from build123d import *

# Parameters (mm, degrees)
SKETCH_1_W      = 200
SKETCH_1_H      = 200
EXTRUDE_1_DEPTH = 150
SKETCH_2_R      = 40
EXTRUDE_2_DEPTH = 10
EXTRUDE_START   = 10
SKETCH_3_R      = 40
EXTRUDE_3_DEPTH = 10


with BuildPart() as part:
    # 草图1 → 凸台-拉伸1 (new, symmetric)
    with BuildSketch(Plane.XY):
        Rectangle(SKETCH_1_W, SKETCH_1_H)
    extrude(amount=EXTRUDE_1_DEPTH, both=True)

    # 草图2 → 凸台-拉伸2 (add)
    with BuildSketch(Plane.XY.offset(150)):
        Circle(SKETCH_2_R)
    extrude(amount=EXTRUDE_2_DEPTH)

    # 草图3 → 凸台-拉伸3 (add)
    with BuildSketch(Plane(origin=(0, 0, -150), x_dir=(-1, 0, 0), z_dir=(0, 0, -1)).offset(EXTRUDE_START)):
        with Locations(Location((0, 0, 0), (0, 0, 180))):
            Circle(SKETCH_3_R)
    extrude(amount=-EXTRUDE_3_DEPTH)


solid = part.part
Design review of the part built by this model. Coordinates are the model's own, in mm. A direction names the side the tool comes from. Round coordinates to 2 decimals unless told otherwise and drop trailing zeros. Write each loop counter-clockwise with the first axis right and the second up, starting at its lowest first coordinate (ties: lowest second). Pieces come first, ordered by that corner, then holes. Notation, with made-up numbers: (-31, 36.5) - (-14, 36.5) arc R9 ccw to (-14, 47.5) - close; hole circle Ø8 at (46.5, 69). An arc over 180 degrees is marked (long way). Use a Markdown table: item, result. Add a question column.
1. We need section C-C (x = 51.5). State the section outline as (y, z) points.
2. For faces 1 (the face through (-1, 46, -150)), 2 (the face through (-1, -1, -160)), 3 (the face through (-8.67, -39.05, 154.93)), list the 3-axis set-ups (+Z, -Z, +X, -X, +Y, -Y) from which the entire face can be reached by the end or side of a thin tool; tool diameter is ignored.
3. Clearance check with flat-ended pins moving along their axes: pin 1 (12 mm diameter, centred on x = 10.5, y = 60, fed in from -Z); pin 2 (1.5 mm diameter, centred on x = -47, y = 58.5, fed in from +Z). State where each tip first meets the part, or that it passes through.
4. We need section A-A (x = 0). State the section outline as (y, z) points.
5. Wall thickness on probe 1 along Z at (x, y) = (69, -30.5): over which ranges is the line inside the solid? List them lowest first.
Output:
| question | item | result |
|---|---|---|
| 1 | outline | (-100, -150) - (100, -150) - (100, 150) - (-100, 150) - close |
| 2 | face 1 | -Z |
| 2 | face 2 | -Z, +X, -X, +Y, -Y |
| 2 | face 3 | +Z |
| 3 | pin 1 | stops at z = -150 |
| 3 | pin 2 | stops at z = 150 |
| 4 | outline | (-100, -150) - (-40, -150) - (-40, -160) - (40, -160) - (40, -150) - (100, -150) - (100, 150) - (40, 150) - (40, 160) - (-40, 160) - (-40, 150) - (-100, 150) - close |
| 5 | probe 1 | z = -150 to 150 |
